Drawing for the job (mm, zero at the part's lowest x, y, z). Coordinates: 2 decimals unless noted, no trailing zeros. Order: outer loops, then holes, each group sorted by start corner. A loop starts at its lowest first (then second) coordinate and runs counter-clockwise, first axis right, second up.
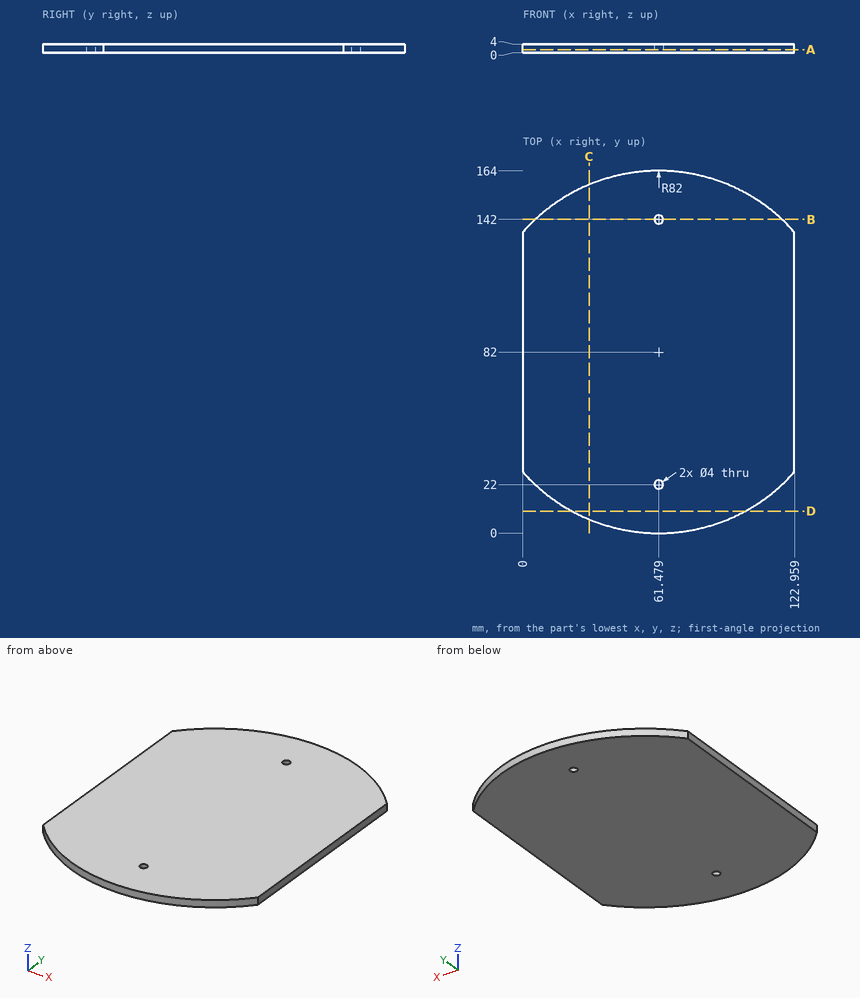
1) Slice it at B-B (y = 142). List the corners of the cut face in (x, z).
2) Slice it at D-D (y = 10). List the corners of the cut face in (x, z).
3) Pin check, flat tip, straight feed: P1, Ø1.5, axis at x = 100.5, z = 1.5, coming from the -Y side. Stop position of the tip, or through.
4) Drill centre lines: probe 1 along Y at (x, z) = (62, 2.2); probe 2 along X at (y, z) = (142, 1.3) (1 decimal); probe 3 along Y at (x, z) = (40.5, 3.05). Where is each one in solid material? Low to high.
5) Slice it at C-C (x = 30). List the corners of the cut face in (y, z).
6) Slice it at A-A (z = 1.4). List the corners of the cut face in (x, y).
Worked out:
1. outline: (5.59, 0) - (59.48, 0) - (59.48, 4) - (5.59, 4) - close; (63.48, 0) - (117.37, 0) - (117.37, 4) - (63.48, 4) - close
2. outline: (22.24, 0) - (100.72, 0) - (100.72, 4) - (22.24, 4) - close
3. P1: stops at y = 9.48
4. probe 1: y = 0 to 20.07, 23.93 to 140.07, 143.93 to 164
4. probe 2: x = 5.6 to 59.5, 63.5 to 117.4
4. probe 3: y = 2.73 to 161.27
5. outline: (6.28, 0) - (157.72, 0) - (157.72, 4) - (6.28, 4) - close
6. outline: (0, 27.74) arc R82 ccw to (122.96, 27.74) - (122.96, 136.26) arc R82 ccw to (0, 136.26) - close; hole circle Ø4 at (61.48, 22); hole circle Ø4 at (61.48, 142)
